Verification items for the finished model (mm, model axes). Face numbers are marked on the shaded views. Round coordinates to 2 decimals unless told otherwise and drop trailing zeros. Order: outer loops, then holes, each group sorted by start corner. A loop starts at its lowest first (then second) coordinate and runs counter-clockwise, first axis right, second up. Notation, with made-up numbers: M 71,66 L 100,66 A8 cw 100,81 Z; hole C 66,13.5 d9. An arc over 180 degrees is marked long. Return JSON: item names as keys, results as strings. Group by question number.
Autodesk Inventor part; units mm, degrees
ref_plane "YZ Plane" through (0, 0, 0) normal (1, 0, 0) x (0, 1, 0)
ref_plane "XZ Plane" through (0, 0, 0) normal (0, 1, 0) x (-1, 0, 0)
ref_plane "XY Plane" through (0, 0, 0) normal (0, 0, 1) x (1, 0, 0)
sketch "Sketch1" plane through (0, 0, 0) normal (0, 1, 0) x (-1, 0, 0)
  line L0 (0, 0) -> (220.218, 0)
  line L1 (220.218, 0) -> (220.218, -267.97)
  line L2 (220.218, -267.97) -> (0, -267.97)
  line L3 (0, -267.97) -> (0, 0)
  circle A0 centre (110.109, -133.985) radius 57.15
  circle A1 centre (110.109, -133.985) radius 50.8
  line L4 (220.218, 0) -> (220.218, -25.4)
  circle A2 centre (201.168, -248.92) radius 9.525
  circle A3 centre (201.168, -19.05) radius 9.525
  circle A4 centre (19.05, -248.92) radius 9.525
  circle A5 centre (19.05, -19.05) radius 9.525
  line L5 (181.0385, -172.085) -> (193.7385, -172.085)
  line L6 (193.7385, -172.085) -> (206.4385, -172.085)
  line L7 (181.0385, -172.085) -> (206.4385, -172.085)
  line L8 (206.4385, -172.085) -> (206.4385, -159.385)
  line L9 (206.4385, -159.385) -> (181.0385, -159.385)
  line L10 (181.0385, -95.885) -> (193.7385, -95.885)
  line L11 (193.7385, -95.885) -> (206.4385, -95.885)
  line L12 (181.0385, -95.885) -> (206.4385, -95.885)
  line L13 (206.4385, -95.885) -> (206.4385, -108.585)
  line L14 (206.4385, -108.585) -> (181.0385, -108.585)
  line L15 (181.0385, -172.085) -> (181.0385, -159.385)
  line L16 (181.0385, -108.585) -> (181.0385, -95.885)
  circle A6 centre (171.8873, -209.1593) radius 34.925
  circle A7 centre (48.3307, -209.1593) radius 34.925
  circle A8 centre (171.8873, -58.8107) radius 34.925
  circle A9 centre (48.3307, -58.8107) radius 34.925
  circle A10 centre (171.8873, -58.8107) radius 9.525
  circle A11 centre (171.8873, -209.1593) radius 9.525
  circle A12 centre (48.3307, -209.1593) radius 9.525
  circle A13 centre (48.3307, -58.8107) radius 9.525
  dimension "d0" = 220.218
  dimension "d1" = 267.97
  dimension "d41" = 12.7
  dimension "d44" = 12.7
  dimension "d52" = 69.85
  dimension "d53" = 19.05
  dimension "d54" = 19.05
  dimension "d57" = 19.05
  dimension "d58" = 19.05
extrude "Extrusion3" add sketch "Sketch1" along normal blind 40.64 contours L0 L1 L2 L3 | A0 | A1 | A2 | A3 | A4 | A5 | L15 L9 L8 L6 L5 | L10 L11 L13 L14 L16 | A6 | A7 | A8 | A9 | A10 | A11 | A12 | A13
extrude "Extrusion4" cut sketch "Sketch1" along normal blind 40.64 contours A1
extrude "Extrusion5" cut sketch "Sketch1" along normal blind 12.7 contours A0 | A1
sketch "Sketch3" plane through (0, 40.64, 0) normal (0, 1, 0) x (1, 0, 0)
  line L0 (0, 267.97) -> (-220.218, 267.97)
  line L1 (-220.218, 0) -> (0, 0)
  circle A0 centre (-110.109, 133.985) radius 57.15
  dimension "d21" = 114.3
extrude "Extrusion6" cut sketch "Sketch3" against normal blind 3.175
extrude "Extrusion8" cut sketch "Sketch1" along normal blind 87.3125 contours A2 | A3 | A4 | A5
extrude "Extrusion9" add sketch "Sketch1" against normal blind 25.4 contours L15 L9 L8 L6 L5 | L10 L11 L13 L14 L16
fillet "Fillet1" radius 12.7 4 edges at (-181.0385, -25.4, -102.235) (-181.0385, -25.4, -165.735) (-206.4385, -25.4, -165.735) (-206.4385, -25.4, -102.235)
sketch "Sketch4" plane through (-206.4385, 0, -95.885) normal (0, 0, 1) x (1, 0, 0)
  arc A0 (0, -12.7) -> (25.4, -12.7) centre (12.7, -12.7) ccw
  circle A1 centre (12.7, -12.7) radius 6.35
  point P0 (206.4385, 0)
  dimension "d48" = 12.7
extrude "Extrusion10" cut sketch "Sketch4" along normal mid plane 436.5625
extrude "Extrusion11" cut sketch "Sketch1" along normal blind 125.4125 contours A10 | A11 | A12 | A13
properties part number "Wash_Base_Bottom"
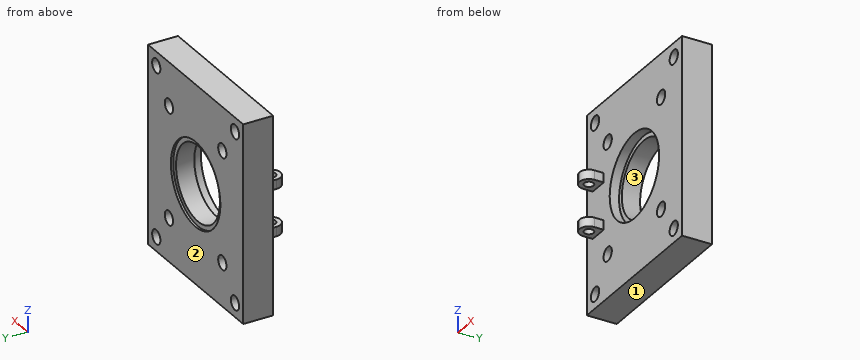
1. Thickness scan on line 1 along X through (y, z) = (13, -252.5); line 2 along X through (y, z) = (6.5, -207); line 3 along Y through (x, z) = (-190, -27). Record the ranges inside material, lowest first. Write a range as from..to.
2. Draft check along Z on the marked faces 1, 2 and 3. Enter one of: +Z half, -Z half, draft (parallel to the pull), parting line (faces both ways), or undercut.
3. Cross-section at B-B (z = -248.92). Enter the section's corners in (x, y) (3 decimals), plus the area to 3 significant figures.
4. Go/stop test with flat-tipped pins: pin 1 (10 mm diameter, centred on y = -8.5, z = -103.5, fed in from -X); pin 2 (1.5 mm diameter, centred on x = -133.5, z = -35, fed in from -Y); pin 3 (16.5 mm diameter, centred on x = -193.74, y = -12.7, fed in from -Z) (3 decimals). Record where each tip stops, or that it passes through.
5. Cross-section at A-A (x = -19.05). Enter the section's corners in (y, z) (3 decimals).
6. Cross-section at C-C (y = 9). Give the number of separate pieces and of enclosed holes in the cut face, plus the area to 3 significant figures.
7. Cross-section at D-D (z = -156). Enter the section's corners in (x, y) (3 decimals).
Computed:
{
 "1": {"line 1": "x = -220.22..-209.99, -192.34..-27.88, -10.22..0", "line 2": "x = -220.22..-181.16, -162.61..-57.61, -39.05..0", "line 3": "y = 0..40.64"},
 "2": {"face 1": "-Z half", "face 2": "draft", "face 3": "undercut"},
 "3": {"outline": "M -220.218,0 L -210.693,0 L -210.693,40.64 L -220.218,40.64 Z; M -191.643,0 L -28.575,0 L -28.575,40.64 L -191.643,40.64 Z; M -9.525,0 L 0,0 L 0,40.64 L -9.525,40.64 Z", "area": "7,400 mm²"},
 "4": {"pin 1": "stops at x = -206.44", "pin 2": "stops at y = 0", "pin 3": "stops at z = -172.085"},
 "5": {"outline": "M 0,-267.97 L 40.64,-267.97 L 40.64,-258.445 L 0,-258.445 Z; M 0,-239.395 L 40.64,-239.395 L 40.64,-28.575 L 0,-28.575 Z; M 0,-9.525 L 40.64,-9.525 L 40.64,0 L 0,0 Z"},
 "6": {"separate pieces": "1", "enclosed holes": "9", "area": "46,500 mm²"},
 "7": {"outline": "M -220.218,0 L -162.849,0 L -162.849,12.7 L -155.891,12.7 L -155.891,37.465 L -162.849,37.465 L -162.849,40.64 L -220.218,40.64 Z; M -64.327,12.7 L -57.369,12.7 L -57.369,0 L 0,0 L 0,40.64 L -57.369,40.64 L -57.369,37.465 L -64.327,37.465 Z"}
}
